```python
from build123d import *

# Parameters (mm, degrees)
F0_W     = 45
F0_H     = 45
F1_DEPTH = 2.5
F2_SIZE  = 10.5
F4_DEPTH = 2.5
F5_R     = 2
F3_R     = 4.3
F6_DEPTH = 25
F8_DEPTH = 2.5


with BuildPart() as f1:
    # F0 (on Front) → F1 (new body)
    with BuildSketch(Plane.XZ):
        Rectangle(F0_W, F0_H)
    extrude(amount=F1_DEPTH)

    # F2
    f2_edges = [f1.edges().sort_by_distance(p)[0] for p in [
        (-22.5, -1.25, 22.5),
        (22.5, -1.25, 22.5),
    ]]
    chamfer(f2_edges, length=F2_SIZE)

    # F3 (on face) → F4 (join)
    with BuildSketch(Plane.XZ.offset(2.5)):
        Polygon((-17.5, -22.5), (-17.5, 9.928932), (-9.928932, 17.5), (9.928932, 17.5), (17.5, 9.928932), (17.5, -22.5), (22.5, -22.5), (22.5, 12), (12, 22.5), (-12, 22.5), (-22.5, 12), (-22.5, -22.5), align=None)
    extrude(amount=F4_DEPTH)

    # F5
    f5_edges = [f1.edges().sort_by_distance(p)[0] for p in [
        (22.5, 0, -5.25),
        (17.25, 0, 17.25),
        (0, 0, -22.5),
        (0, 0, 22.5),
        (-22.5, 0, -5.25),
        (-17.25, 0, 17.25),
    ]]
    fillet(f5_edges, radius=F5_R)

    # F3 (on face) → F6 (cut)
    with BuildSketch(Plane.XZ.offset(2.5)):
        Circle(F3_R)
    extrude(amount=-F6_DEPTH, mode=Mode.SUBTRACT)

    # F7 (on face) → F8 (cut)
    with BuildSketch(Plane.XZ.offset(5)):
        with BuildLine():
            Line((20, -20), (18.5, -20))
            ThreePointArc((18.5, -20), (18.93934, -21.06066), (20, -21.5))
            Line((20, -21.5), (20, -20))
        make_face()
        with BuildLine():
            ThreePointArc((21.5, -20), (20, -18.5), (18.5, -20))
            Line((18.5, -20), (20, -20))
            Line((20, -20), (20, -21.5))
            ThreePointArc((20, -21.5), (21.06066, -21.06066), (21.5, -20))
        make_face()
        with BuildLine():
            ThreePointArc((-21.5, -20), (-21.06066, -21.06066), (-20, -21.5))
            Line((-20, -21.5), (-20, -20))
            Line((-20, -20), (-21.5, -20))
        make_face()
        with BuildLine():
            Line((-20, -20), (-20, -21.5))
            ThreePointArc((-20, -21.5), (-18.93934, -21.06066), (-18.5, -20))
            ThreePointArc((-18.5, -20), (-20, -18.5), (-21.5, -20))
            Line((-21.5, -20), (-20, -20))
        make_face()
        with BuildLine():
            ThreePointArc((-20, 8.428932), (-18.93934, 8.868272), (-18.5, 9.928932))
            Line((-18.5, 9.928932), (-20, 9.928932))
            Line((-20, 9.928932), (-20, 8.428932))
        make_face()
        with BuildLine():
            Line((-20, 9.928932), (-18.5, 9.928932))
            ThreePointArc((-18.5, 9.928932), (-21.06066, 10.989592), (-20, 8.428932))
            Line((-20, 8.428932), (-20, 9.928932))
        make_face()
        with BuildLine():
            ThreePointArc((1.5, 20), (-1.06066, 21.06066), (0, 18.5))
            ThreePointArc((0, 18.5), (1.06066, 18.93934), (1.5, 20))
        make_face()
        with BuildLine():
            Line((20, 9.928932), (18.5, 9.928932))
            ThreePointArc((18.5, 9.928932), (18.93934, 8.868272), (20, 8.428932))
            Line((20, 8.428932), (20, 9.928932))
        make_face()
        with BuildLine():
            ThreePointArc((21.5, 9.928932), (20, 11.428932), (18.5, 9.928932))
            Line((18.5, 9.928932), (20, 9.928932))
            Line((20, 9.928932), (20, 8.428932))
            ThreePointArc((20, 8.428932), (21.06066, 8.868272), (21.5, 9.928932))
        make_face()
    extrude(amount=-F8_DEPTH, mode=Mode.SUBTRACT)


solid = f1.part
```
Model file for the job. Use its own axes, mm. A direction names the side the tool comes from. Coordinates: 2 decimals unless noted, no trailing zeros. Loops run counter-clockwise (first coordinate to the right, second up) from the corner with the lowest first, then second, coordinate; pieces in that order, holes last. Notation, with made-up numbers: (18.25, 17.25) - (22.25, 17.25) arc R9 ccw to (22.25, 23.25) - close; hole circle Ø5 at (17, -8). An arc over 180 degrees is marked (long way). Answer as a JSON object with one key per item and string values. Group by question number.
(1) Cut at C-C (x = 6). Give the cut face in (y, z), then the cut area to 3 significant figures.
(2) Cut at B-B (y = -0.9). Give the cut face in (x, z), then the cut area to 3 significant figures.
(3) Two-plate mould, pull along Z, no slides. Class faces 4 (the face through (0, -4, 17.5)), 5 (the face through (-22.5, -3, -5)), 6 (the face through (0, -2.5, 20)): released by +Z, released by -Z, zero draft, split by the parting line, or undercut.
(4) Cut at D-D (z = -15). Give the cut face in (x, y), then the cut area to 3 significant figures.
(5) Flat gauge pins, fed straight in: pin 1 (2 mm diameter, centred on x = -4, y = -4.5, fed in from -Z); pin 2 (0.9 mm diameter, centred on x = -19.5, z = 10.5, fed in from -Y). Where does each tip first touch, or does it go through?
(6) Tool access for faces 1 (the face through (0.17, -0.57, 21.9)), 2 (the face through (-20, -2.5, -20)), 3 (the face through (0, -2.5, -7)): list every direction of +Z, -Z, +X, -X, +Y, -Y with a clear straight run to the whole face (end or side of a thin tool).
(7) Cut at A-A (z = 0). Give the cut face in (x, y).
(8) Probe line 1 along X through (y, z) = (-3.05, 1); line 2 along Z through (x, y) = (-20, -4.2); line 3 along Z through (x, y) = (0, -3.3). List the from-to ranges inside material, lowest first.
Geometry says:
{
 "1": {"outline": "(-5, 17.5) - (-2.5, 17.5) - (-2.5, -22.5) - (-2, -22.5) arc R2 ccw to (0, -20.5) - (0, 20.5) arc R2 ccw to (-2, 22.5) - (-5, 22.5) - close", "area": "123 mm^2"},
 "2": {"outline": "(-22.17, -22.17) - (22.17, -22.17) - (22.17, 11.86) - (11.86, 22.17) - (-11.86, 22.17) - (-22.17, 11.86) - close; hole circle Ø8.6 at (0, 0)", "area": "1,800 mm^2"},
 "3": {"face 4": "released by -Z", "face 5": "zero draft", "face 6": "undercut"},
 "4": {"outline": "(-22.5, -5) - (-17.5, -5) - (-17.5, -2.5) - (17.5, -2.5) - (17.5, -5) - (22.5, -5) - (22.5, -2) arc R2 ccw to (20.5, 0) - (-20.5, 0) arc R2 ccw to (-22.5, -2) - close", "area": "136 mm^2"},
 "5": {"pin 1": "stops at z = 17.5", "pin 2": "stops at y = -2.5"},
 "6": {"face 1": "+Z, +X, -X, +Y", "face 2": "-Y", "face 3": "-Z, -Y"},
 "7": {"outline": "(-22.5, -5) - (-17.5, -5) - (-17.5, -2.5) - (-4.3, -2.5) - (-4.3, 0) - (-20.5, 0) arc R2 ccw to (-22.5, -2) - close; (4.3, -2.5) - (17.5, -2.5) - (17.5, -5) - (22.5, -5) - (22.5, -2) arc R2 ccw to (20.5, 0) - (4.3, 0) - close"},
 "8": {"line 1": "x = -22.5 to -17.5, 17.5 to 22.5", "line 2": "z = -22.5 to -21.5, -18.5 to 8.43, 11.43 to 14.5", "line 3": "z = 17.5 to 18.5, 21.5 to 22.5"}
}
